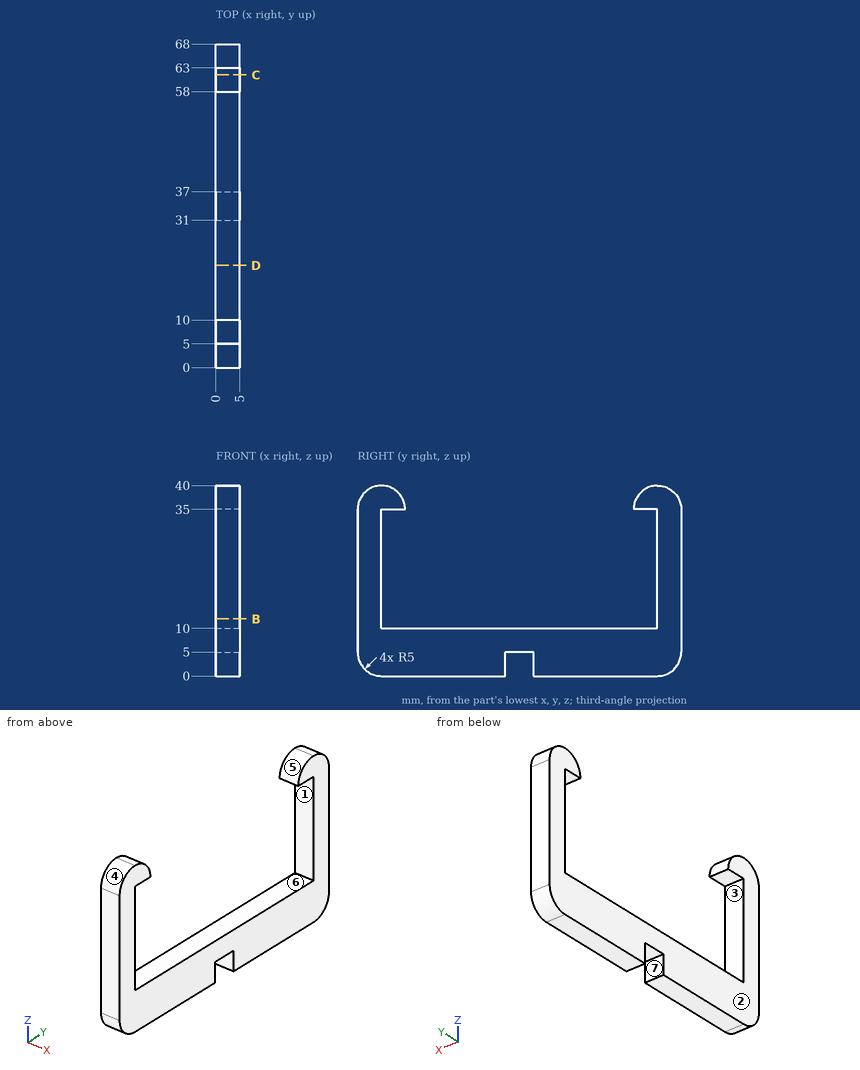
Input: dimensioned drawing with shaded views. Units: mm. Origin: part minimum x, y, z. A direction names the side the tool comes from. Coordinates: 2 decimals unless noted, no trailing zeros. Loops run counter-clockwise (first coordinate to the right, second up) from the corner with the lowest first, then second, coordinate; pieces in that order, holes last. Notation, with made-up numbers: M 73.5,15 L 106.5,15 A20 cw 106.5,28 Z; hole C 7.5,45.25 d7. An arc over 180 degrees is marked long. Use a Markdown table: item, result. Add a question column.
Q1. Material intervals for L1, parallel to Y at x = 1.1, z = 15.5; L2, parallel to Z at x = 2.85, y = 12; L3, parallel to Z at x = 4.75, y = 59, sorted ascending.
Q2. Section query C-C, the plane y = 61.5. Return loops of the section in (x, z).
Q3. Section query D-D, the plane y = 21.5. Return loops of the section in (x, z).
Q4. Section query B-B, the plane z = 12. Return loops of the section in (x, y).
Q5. Draft query along Y for the marked faces 1, 2, 3 and 4. Return one class per face: pulls with the +Y half, pulls with the -Y half, needs draft (parallel to the pull), parting line crosses it, or undercut.
Q6. First-contact query: pin 1 (2.5 mm diameter, centred on x = 3.5, z = 2.5, fed in from +Y); pin 2 (1.5 mm diameter, centred on x = 3, z = 3.5, fed in from -Y). Flat tips, straight axial feed; report the tip coordinate or a pass-through.
Q7. Access query for the marked faces 5, 6 and 7. Directions: +Z, -Z, +X, -X, +Y, -Y. A direction counts if a zero-diameter tool reaches every point of the face in a straight line with its end or side. Return the directions, or none.
Result:
| question | item | result |
|---|---|---|
| 1 | L1 | y = 0 to 5, 63 to 68 |
| 1 | L2 | z = 0 to 10 |
| 1 | L3 | z = 0 to 10, 35 to 38 |
| 2 | outline | M 0,0 L 5,0 L 5,10 L 0,10 Z; M 0,35 L 5,35 L 5,39.77 L 0,39.77 Z |
| 3 | outline | M 0,0 L 5,0 L 5,10 L 0,10 Z |
| 4 | outline | M 0,0 L 5,0 L 5,5 L 0,5 Z; M 0,63 L 5,63 L 5,68 L 0,68 Z |
| 5 | face 1 | undercut |
| 5 | face 2 | needs draft |
| 5 | face 3 | undercut |
| 5 | face 4 | pulls with the -Y half |
| 6 | pin 1 | stops at y = 67.84 |
| 6 | pin 2 | stops at y = 0.06 |
| 7 | face 5 | +Z, +X, -X |
| 7 | face 6 | +X, -X |
| 7 | face 7 | -Z, +X, -X |
